Can you work these out from the model? Positions are in its coordinate system, mm. Face numbers are marked on the shaded views. A direction names the side the tool comes from. Coordinates: 2 decimals unless noted, no trailing zeros. Loops run counter-clockwise (first coordinate to the right, second up) from the corner with the lowest first, then second, coordinate; pieces in that order, holes last. Notation, with made-up numbers: M 84,35 L 133,35 A21 cw 133,66 Z; hole C -25,35.5 d5. An arc over 180 degrees is marked long. Answer as a JSON object with one key per item and string values. Group by question number.
Item 1: We'd pull the mould along X, two halves only. Please class the marked faces 1, 2 and 3: +X half, -X half, draft (parallel to the pull), parting line (faces both ways), or undercut.
Item 2: Suppose I cut it at B-B (z = 13.5). Write out the boundary of the cut face in (x, y).
Item 3: If I drill on line 1 (X direction, y = -6, z = -12); line 2 (X direction, y = -3.25, z = -12); line 3 (Y direction, x = 78.5, z = -16), over which ranges is the centre line in solid material (lowest first)?
Item 4: Which directions (+Z, -Z, +X, -X, +Y, -Y) give clear straight access to the entire face, cutting with the end or side of a thin tool? Please do the marked faces 4 and 5.
Item 5: Suppose I cut it at A-A (z = -19). Write out the boundary of the cut face in (x, y), then the cut area to 3 significant figures.
Item 6: Suppose I cut it at C-C (x = 64). Write out the boundary of the cut face in (y, z), then the cut area to 3 significant figures.
Item 7: I'm going to push flat-ended pins straight in: pin 1 Ø13 at (x, z) = (70.41, -12) entering from +Y; pin 2 Ø8 at (x, z) = (90, -19) entering from +Y. Where does each tip first touch, or does it pass through?
Item 8: Suppose I cut it at D-D (x = 98). Write out the boundary of the cut face in (y, z), then the cut area to 3 significant figures.
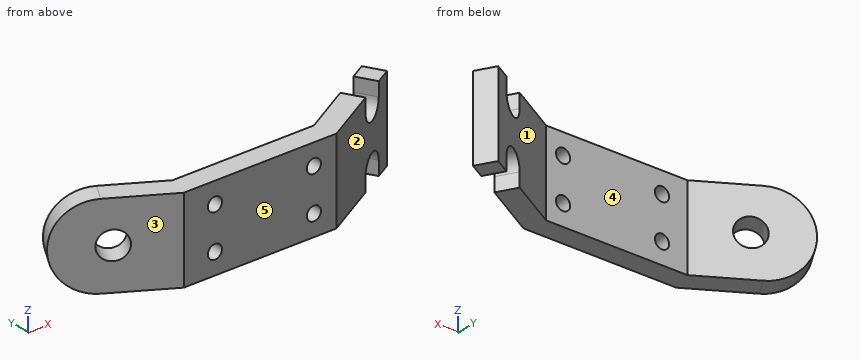
```python
from build123d import *

# Parameters (mm, degrees)
EXTRUDE_1_DEPTH     = 24
FILLET_1_RADIUS     = 24
FILLET_1_LENGTH     = 12
SKETCH_3_R          = 8
CUT_EXTRUDE_2_DEPTH = 142.334600959
SKETCH_4_R          = 4
CUT_EXTRUDE_3_DEPTH = 142.334600959
CUT_EXTRUDE_4_DEPTH = 135.667997045


with BuildPart() as part:
    # 草圖1 → 伸長-薄件1 (new, symmetric)
    with BuildSketch(Plane.XY):
        Polygon((130.229473419, 29), (80, 0), (0, 0), (-50.229473419, 29), (-56.229473419, 18.607695155), (-3.215390309, -12), (83.215390309, -12), (136.229473419, 18.607695155), align=None)
    extrude(amount=EXTRUDE_1_DEPTH, both=True)

    # 圓角1: full round fillet: the end face becomes a half cylinder, R = half its width
    fillet_1_face = Plane((-53.229473419, 23.803847577, 0), x_dir=(0.5, 0.866025403784, 0), z_dir=(-0.866025403784, 0.5, 0))  # on the end face: x along it, z out of the body
    fillet_1_slab = fillet_1_face.offset(-FILLET_1_RADIUS / 2) * Box(FILLET_1_LENGTH, 2 * FILLET_1_RADIUS, FILLET_1_RADIUS, mode=Mode.PRIVATE)  # the body's end, R deep
    fillet_1_round = Plane((-32.444863728, 11.803847577, 0), x_dir=(-0.866025403784, 0.5, 0), z_dir=(0.5, 0.866025403784, 0)) * Cylinder(FILLET_1_RADIUS, FILLET_1_LENGTH, mode=Mode.PRIVATE)  # its axis R under the face
    add(fillet_1_slab - fillet_1_round, mode=Mode.SUBTRACT)

    # 草圖3 → 除料-伸長2 (cut, through all)
    with BuildSketch(Plane(origin=(0, 0, 0), x_dir=(0.8660254037844416, -0.49999999999999484, 0), z_dir=(0.49999999999999484, 0.8660254037844416, 0))):
        with Locations(Location((-28.36733721, 0, 0), (0, 0, 180))):
            Circle(SKETCH_3_R)
    extrude(amount=-CUT_EXTRUDE_2_DEPTH, mode=Mode.SUBTRACT)

    # 草圖4 → 除料-伸長3 (cut, through all)
    with BuildSketch(Plane(origin=(0, 0, 0), x_dir=(1, 0, 0), z_dir=(0, 1, 0))):
        with Locations(Location((14.406554247, -12, 0), (0, 0, 270))):
            Circle(SKETCH_4_R)
        with Locations(Location((70.406554247, -12, 0), (0, 0, 270))):
            Circle(SKETCH_4_R)
        with Locations(Location((70.406554247, 12, 0), (0, 0, 90))):
            Circle(SKETCH_4_R)
        with Locations(Location((14.406554247, 12, 0), (0, 0, 90))):
            Circle(SKETCH_4_R)
    extrude(amount=-CUT_EXTRUDE_3_DEPTH, mode=Mode.SUBTRACT)

    # 草圖5 → 除料-伸長4 (cut, through all)
    with BuildSketch(Plane(origin=(20, -34.641016151, 0), x_dir=(0.866025403784438, 0.500000000000001, 0), z_dir=(-0.500000000000001, 0.866025403784438, 0))):
        with BuildLine():
            Line((101.282032303, -24), (101.282032303, -16))
            ThreePointArc((101.282032303, -16), (109.282032303, -8), (117.282032303, -16))
            Line((117.282032303, -16), (117.282032303, -24))
            Line((117.282032303, -24), (101.282032303, -24))
        make_face()
        with BuildLine():
            Line((117.282032303, 24), (101.282032303, 24))
            Line((101.282032303, 24), (101.282032303, 16))
            ThreePointArc((101.282032303, 16), (109.282032303, 8), (117.282032303, 16))
            Line((117.282032303, 16), (117.282032303, 24))
        make_face()
    extrude(amount=-CUT_EXTRUDE_4_DEPTH, mode=Mode.SUBTRACT)


solid = part.part
```
From the geometry:
{
 "1": {"face 1": "undercut", "face 2": "+X half", "face 3": "-X half"},
 "2": {"outline": "M -52.63,16.53 L -3.22,-12 L 10.7,-12 L 10.7,0 L 0,0 L -46.63,26.92 Z; M 18.11,-12 L 66.7,-12 L 66.7,0 L 18.11,0 Z; M 74.11,-12 L 83.22,-12 L 114.06,5.81 L 108.06,16.2 L 80,0 L 74.11,0 Z; M 121.22,23.8 L 127.22,13.41 L 136.23,18.61 L 130.23,29 Z"},
 "3": {"line 1": "-13.61 to 10.41, 18.41 to 66.41, 74.41 to 93.61", "line 2": "-18.37 to 10.41, 18.41 to 66.41, 74.41 to 98.37", "line 3": "-12 to 0"},
 "4": {"face 4": "+Z, -Z, +Y", "face 5": "+Z, -Z, +X, -X, -Y"},
 "5": {"outline": "M -48.14,13.94 L -3.22,-12 L 83.22,-12 L 113.71,5.61 L 107.71,16 L 80,0 L 0,0 L -42.14,24.33 Z; M 121.57,24 L 127.57,13.61 L 136.23,18.61 L 130.23,29 Z", "area": "2,130 mm2"},
 "6": {"outline": "M -12,-24 L 0,-24 L 0,24 L -12,24 Z", "area": "576 mm2"},
 "7": {"pin 1": "y = 0", "pin 2": "y = 8.08"},
 "8": {"outline": "M -3.46,-24 L 10.39,-24 L 10.39,24 L -3.46,24 Z", "area": "665 mm2"}
}
